Here's how the part is built. I have some questions about the finished solid (model axes, mm). Face numbers are marked on the shaded views. A direction names the side the tool comes from. Coordinates: 2 decimals unless noted, no trailing zeros. Write each loop counter-clockwise with the first axis right and the second up, starting at its lowest first coordinate (ties: lowest second). Pieces come first, ordered by that corner, then holes.
(1) Please list where these lines run through material, in increasing order: probe 1 along Z at (x, y) = (11, 2.65); probe 2 along Y at (x, z) = (7, 3.45); probe 3 along X at (y, z) = (17, 3.85).
(2) Imagine slicing it at B-B, the plane x = 17.75. List the corners of the cut face in (y, z) for me, plus the area to 3 significant figures.
(3) Imagine slicing it at A-A, the plane y = 37. List the corners of the cut face in (x, z) for me, plus the area to 3 significant figures.
(4) Imagine slicing it at D-D, the plane z = 0.6. List the corners of the cut face in (x, y) for me, plus the area to 3 significant figures.
(5) Thinking about a two-plate mould opening in Y: for the marked faces 1, 2 and 3, which applies, released by +Y, released by -Y, zero draft, split by the parting line, or undercut?
(6) For pin 1 Ø12 at (x, y) = (19.5, 9.5) entering from -Z; pin 2 Ø0.5 at (x, z) = (18, 3.5) entering from -Y; pin 3 Ø1.1 at (x, z) = (22.5, 2.5) entering from -Y, each with a flat end and sliding along its axis, tell me the tip position at first contact or that it passes through.
(7) Which directions (+Z, -Z, +X, -X, +Y, -Y) give clear straight access to the entire face, cutting with the end or side of a thin tool? Please do the marked faces 4, 5 and 6.
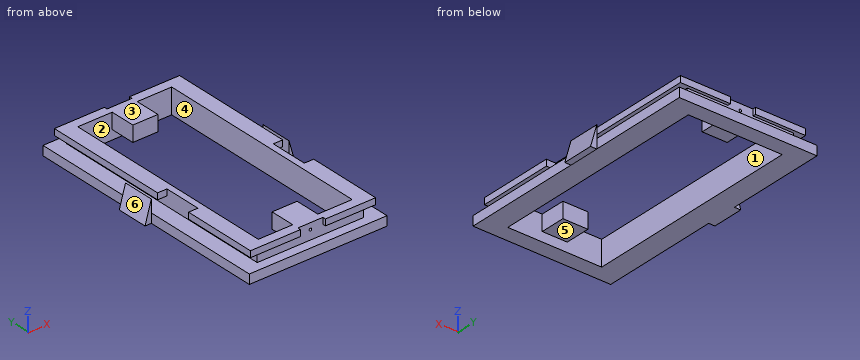
```python
from build123d import *

# Parameters (mm, degrees)
CYLINDER_R             = 0.2
CYLINDER_DEPTH         = 4
CYLINDER_ROLL_ANGLE    = 90
CYLINDER001_R          = 0.2
CYLINDER001_DEPTH      = 4
CYLINDER001_ROLL_ANGLE = 90
BOX010_W               = 4
BOX010_H               = 2
BOX010_DEPTH           = 2.5
BOX011_W               = 4
BOX011_H               = 2
BOX011_DEPTH           = 2.5
BOX007_W               = 6
BOX007_H               = 6
BOX007_DEPTH           = 5
BOX006_W               = 6
BOX006_H               = 6
BOX006_DEPTH           = 5
BOX001_W               = 15
BOX001_H               = 35
BOX001_DEPTH           = 10
BOX004_W               = 17
BOX004_H               = 37
BOX004_DEPTH           = 2.5
BOX005_W               = 20
BOX005_H               = 38
BOX005_DEPTH           = 1
BOX_W                  = 22
BOX_H                  = 40
BOX_DEPTH              = 1.5
PAD_DEPTH              = 5
PAD001_DEPTH           = 5
BOX008_W               = 4
BOX008_H               = 5
BOX008_DEPTH           = 2.5
BOX009_W               = 4
BOX009_H               = 5
BOX009_DEPTH           = 2.5


with BuildPart() as m3_hole1:
    # Cylinder → Cylinder (new body)
    with BuildSketch(Plane.XY):
        Circle(CYLINDER_R)
    extrude(amount=CYLINDER_DEPTH)


with BuildPart() as m3_hole1_1:
    # Cylinder roll: moved
    add(m3_hole1.part.rotate(Axis((0, 0, 0), (1, 0, 0)), CYLINDER_ROLL_ANGLE))


with BuildPart() as m3_hole1_2:
    # Cylinder placement: moved
    add(m3_hole1_1.part.moved(Location((11, 5.5, 3))))


with BuildPart() as screw_holes:
    # Cylinder001 → Cylinder001 (new body)
    with BuildSketch(Plane.XY):
        Circle(CYLINDER001_R)
    extrude(amount=CYLINDER001_DEPTH)


with BuildPart() as screw_holes_1:
    # Cylinder001 roll: moved
    add(screw_holes.part.rotate(Axis((0, 0, 0), (1, 0, 0)), CYLINDER001_ROLL_ANGLE))


with BuildPart() as screw_holes_2:
    # Cylinder001 placement: moved
    add(screw_holes_1.part.moved(Location((11, 38.5, 3))))

    # Fusion003: union M3 hole1
    add(m3_hole1_2.part)


with BuildPart() as remove:
    # Box010 → Box010 (new body)
    with BuildSketch(Plane(origin=(9, -0.5, 1.5), x_dir=(1, 0, 0), z_dir=(0, 0, 1))):
        with Locations((2, 1)):
            Rectangle(BOX010_W, BOX010_H)
    extrude(amount=BOX010_DEPTH)


with BuildPart() as fusion004:
    # Box011 → Box011 (new body)
    with BuildSketch(Plane(origin=(9, 38.5, 1.5), x_dir=(1, 0, 0), z_dir=(0, 0, 1))):
        with Locations((2, 1)):
            Rectangle(BOX011_W, BOX011_H)
    extrude(amount=BOX011_DEPTH)

    # Fusion004: union remove
    add(remove.part)


with BuildPart() as space001:
    # Box007 → Box007 (new body)
    with BuildSketch(Plane(origin=(19.5, 13, 1.5), x_dir=(1, 0, 0), z_dir=(0, 0, 1))):
        with Locations((3, 3)):
            Rectangle(BOX007_W, BOX007_H)
    extrude(amount=BOX007_DEPTH)


with BuildPart() as fusion001:
    # Box006 → Box006 (new body)
    with BuildSketch(Plane(origin=(-3.5, 13, 1.5), x_dir=(1, 0, 0), z_dir=(0, 0, 1))):
        with Locations((3, 3)):
            Rectangle(BOX006_W, BOX006_H)
    extrude(amount=BOX006_DEPTH)

    # Fusion001: union space001
    add(space001.part)


with BuildPart() as inner_space:
    # Box001 → Box001 (new body)
    with BuildSketch(Plane(origin=(3.5, 2.5, 0), x_dir=(1, 0, 0), z_dir=(0, 0, 1))):
        with Locations((7.5, 17.5)):
            Rectangle(BOX001_W, BOX001_H)
    extrude(amount=BOX001_DEPTH)


with BuildPart() as track_inner:
    # Box004 → Box004 (new body)
    with BuildSketch(Plane(origin=(2.5, 1.5, 1.5), x_dir=(1, 0, 0), z_dir=(0, 0, 1))):
        with Locations((8.5, 18.5)):
            Rectangle(BOX004_W, BOX004_H)
    extrude(amount=BOX004_DEPTH)


with BuildPart() as track_outer:
    # Box005 → Box005 (new body)
    with BuildSketch(Plane(origin=(1, 1, 3), x_dir=(1, 0, 0), z_dir=(0, 0, 1))):
        with Locations((10, 19)):
            Rectangle(BOX005_W, BOX005_H)
    extrude(amount=BOX005_DEPTH)


with BuildPart() as cut002:
    # Box → Box (new body)
    with BuildSketch(Plane.XY):
        with Locations((11, 20)):
            Rectangle(BOX_W, BOX_H)
    extrude(amount=BOX_DEPTH)

    # Fusion: union track_inner, track_outer
    add(track_inner.part)
    add(track_outer.part)

    # Cut: cut inner space
    add(inner_space.part, mode=Mode.SUBTRACT)

    # Cut001: cut Fusion001
    add(fusion001.part, mode=Mode.SUBTRACT)

    # Cut002: cut Fusion004
    add(fusion004.part, mode=Mode.SUBTRACT)


with BuildPart() as pad:
    # Sketch → Pad (new body)
    with BuildSketch(Plane.XZ.offset(-21)):
        Polygon((0, 0), (0, 3.5), (-1, 0), align=None)
    extrude(amount=PAD_DEPTH)


with BuildPart() as slide_control:
    # Sketch001 → Pad001 (new body)
    with BuildSketch(Plane.XZ.offset(-21)):
        Polygon((21.996317, 3.488174), (21.996317, -0.011826), (22.996317, -0.011826), align=None)
    extrude(amount=PAD001_DEPTH)

    # Fusion005: union Pad
    add(pad.part)


with BuildPart() as slide_control_1:
    # Fusion005 placement: moved
    add(slide_control.part.moved(Location((0, 3, 0))))


with BuildPart() as screw_block1:
    # Box008 → Box008 (new body)
    with BuildSketch(Plane(origin=(9, 1.5, 1.5), x_dir=(1, 0, 0), z_dir=(0, 0, 1))):
        with Locations((2, 2.5)):
            Rectangle(BOX008_W, BOX008_H)
    extrude(amount=BOX008_DEPTH)


with BuildPart() as basesensormount:
    # Box009 → Box009 (new body)
    with BuildSketch(Plane(origin=(9, 33.5, 1.5), x_dir=(1, 0, 0), z_dir=(0, 0, 1))):
        with Locations((2, 2.5)):
            Rectangle(BOX009_W, BOX009_H)
    extrude(amount=BOX009_DEPTH)

    # Fusion002: union screw block1
    add(screw_block1.part)

    # Fusion006: union Cut002, slide control
    add(cut002.part)
    add(slide_control_1.part)

    # Cut003: cut screw holes
    add(screw_holes_2.part, mode=Mode.SUBTRACT)


solid = basesensormount.part
```
Recorded:
1. probe 1: z = 1.5 to 2.8, 3.2 to 4
1. probe 2: y = 1 to 2.5, 37.5 to 39
1. probe 3: x = 2.5 to 3.5, 18.5 to 19.5
2. outline: (0, 0) - (2.5, 0) - (2.5, 4) - (1, 4) - (1, 3) - (1.5, 3) - (1.5, 1.5) - (0, 1.5) - close; (37.5, 0) - (40, 0) - (40, 1.5) - (38.5, 1.5) - (38.5, 3) - (39, 3) - (39, 4) - (37.5, 4) - close
2. area: 13.5 mm2
3. outline: (0, 0) - (3.5, 0) - (3.5, 4) - (1, 4) - (1, 3) - (2.5, 3) - (2.5, 1.5) - (0, 1.5) - close; (9, 1.5) - (13, 1.5) - (13, 4) - (9, 4) - close; (18.5, 0) - (22, 0) - (22, 1.5) - (19.5, 1.5) - (19.5, 3) - (21, 3) - (21, 4) - (18.5, 4) - close; hole circle Ø0.4 at (11, 3)
3. area: 28.4 mm2
4. outline: (-0.83, 19) - (0, 19) - (0, 0) - (22, 0) - (22, 19) - (22.82, 19) - (22.82, 24) - (22, 24) - (22, 40) - (0, 40) - (0, 24) - (-0.83, 24) - close; hole (3.5, 2.5) - (18.5, 2.5) - (18.5, 37.5) - (3.5, 37.5) - close
4. area: 363 mm2
5. face 1: undercut
5. face 2: undercut
5. face 3: zero draft
6. pin 1: stops at z = 0
6. pin 2: stops at y = 1
6. pin 3: stops at y = 19
7. face 4: +Z, -Z
7. face 5: -Z
7. face 6: +Z, -X, +Y, -Y
